```python
from build123d import *

# Parameters (mm, degrees)
BOSS_EXTRUDE1_DEPTH             = 15
H_0_266_DIAMETER_HOLE1_D        = 6.7564
SKETCH5_W                       = 1000
SKETCH5_H                       = 16
SKETCH5_W_2                     = 70
SKETCH5_H_2                     = 20.916111238
CUT_EXTRUDE1_DEPTH              = 243.332416321
BOSS_EXTRUDE4_REACH             = 242.936
SKETCH6_R                       = 3.3782
BOSS_EXTRUDE4_DIRECTION_2_REACH = 242.936


with BuildPart() as part:
    # Sketch1 → Boss-Extrude1 (new, symmetric)
    with BuildSketch(Plane.XY):
        with BuildLine():
            Line((-225, 15), (225, 15))
            ThreePointArc((225, 15), (240, 0), (225, -15))
            Line((225, -15), (-225, -15))
            ThreePointArc((-225, -15), (-240, 0), (-225, 15))
        make_face()
    extrude(amount=BOSS_EXTRUDE1_DEPTH, both=True)

    # H (0.266) Diameter Hole1 (through all)
    with Locations(Plane.XY.offset(15)):
        with Locations((-225, 0), (225, 0)):
            Hole(H_0_266_DIAMETER_HOLE1_D / 2)

    # Sketch5 → Cut-Extrude1 (cut, through all)
    with BuildSketch(Plane(origin=(0, 15, 0), x_dir=(1, 0, 0), z_dir=(0, 1, 0))):
        with Locations((-475, 0)):
            Rectangle(SKETCH5_W, SKETCH5_H)
        with Locations((210, 18.458055619)):
            Rectangle(SKETCH5_W_2, SKETCH5_H_2)
        with Locations((210, -18.458055619)):
            Rectangle(SKETCH5_W_2, SKETCH5_H_2)
    extrude(amount=-CUT_EXTRUDE1_DEPTH, mode=Mode.SUBTRACT)

    # Boss-Extrude4: up to this face of the body (flat: up to its plane)
    boss_extrude4_end = Plane(part.part.faces().sort_by_distance((-30.33914406, 0, 15))[0])
    # Sketch6 → Boss-Extrude4 (add, up to the picked face)
    with BuildSketch(Plane.XY, mode=Mode.PRIVATE) as boss_extrude4_sk1:
        with Locations((225, 0)):
            Circle(SKETCH6_R)
    boss_extrude4_tool1 = split(extrude(boss_extrude4_sk1.sketch, amount=BOSS_EXTRUDE4_REACH, mode=Mode.PRIVATE), bisect_by=boss_extrude4_end, keep=Keep.BOTH, mode=Mode.PRIVATE)
    add(boss_extrude4_tool1.solids().sort_by(Axis((225, 0, 0), (0, 0, 1)))[0])

    # Boss-Extrude4 direction 2: up to this face of the body (flat: up to its plane)
    boss_extrude4_direction_2_end = Plane(part.part.faces().sort_by_distance((-30.33914406, 0, -15))[0])
    # Sketch6 → Boss-Extrude4 direction 2 (add, up to the picked face)
    with BuildSketch(Plane.XY, mode=Mode.PRIVATE) as boss_extrude4_direction_2_sk1:
        with Locations((225, 0)):
            Circle(SKETCH6_R)
    boss_extrude4_direction_2_tool1 = split(extrude(boss_extrude4_direction_2_sk1.sketch, amount=-BOSS_EXTRUDE4_DIRECTION_2_REACH, mode=Mode.PRIVATE), bisect_by=boss_extrude4_direction_2_end, keep=Keep.BOTH, mode=Mode.PRIVATE)
    add(boss_extrude4_direction_2_tool1.solids().sort_by(Axis((225, 0, 0), (0, 0, -1)))[0])


solid = part.part
```
Can you work these out from the model? Positions are in its coordinate system, mm. A direction names the side the tool comes from. Coordinates: 2 decimals unless noted, no trailing zeros. Loops run counter-clockwise (first coordinate to the right, second up) from the corner with the lowest first, then second, coordinate; pieces in that order, holes last.
1) I need wall thicknesses on probe 1 along X at (y, z) = (-0.5, -13.5); probe 2 along Y at (x, z) = (-225, -11.5); probe 3 along Z at (x, y) = (-7, 11). Which ranges of each line are inside material? Lowest first, please.
2) Imagine slicing it at A-A on x = -12. List the corners of the cut face in (y, z) for me.
3) Thinking about a two-plate mould opening in Z: for faces 1 (the flat face through (-109, 0, -8)), 2 (the flat face through (53, -15, 0)), 3 (the flat face through (-30, 0, -15)), which applies, pulls with the +Z half, pulls with the -Z half, needs draft (parallel to the pull), parting line crosses it, or undercut?
4) Which directions (+Z, -Z, +X, -X, +Y, -Y) give clear straight access to the entire face, cutting with the end or side of a thin tool? Please do faces 4 (the flat face through (-30, 0, 15)), 5 (the flat face through (-109, 0, 8)).
5) For pin 1 (3.5 mm diameter, centred on y = -0.5, z = 11, fed in from +X); pin 2 (7.5 mm diameter, centred on y = 5, z = -12.5, fed in from +X); pin 3 (2 mm diameter, centred on x = 186.5, z = -10.5, fed in from +Y); pin 4 (1 mm diameter, centred on y = -11, z = 5, fed in from -X), each with a flat end and sliding along its axis, tell me the tip position at first contact or that it passes through.
6) Imagine slicing it at B-B on y = -8. List the corners of the cut face in (x, z) for me.
7) Imagine slicing it at C-C on z = 4. List the corners of the cut face in (x, y) for me.
8) Imagine slicing it at D-D on y = 9.5. List the corners of the cut face in (x, z) for me, plus the area to 3 significant figures.
Completed:
1. probe 1: x = -239.99 to -228.34, -221.66 to 175, 221.66 to 228.34
1. probe 2: y = -15 to -3.38, 3.38 to 15
1. probe 3: z = -15 to -8, 8 to 15
2. outline: (-15, -15) - (15, -15) - (15, -8) - (-15, -8) - close; (-15, 8) - (15, 8) - (15, 15) - (-15, 15) - close
3. face 1: undercut
3. face 2: needs draft
3. face 3: pulls with the -Z half
4. face 4: +Z, +X, -X, +Y, -Y
4. face 5: -X, +Y, -Y
5. pin 1: stops at x = 228.38
5. pin 2: stops at x = 228.14
5. pin 3: passes through
5. pin 4: stops at x = 25
6. outline: (-237.69, -15) - (175, -15) - (175, -8) - (237.69, -8) - (237.69, 8) - (175, 8) - (175, 15) - (-237.69, 15) - (-237.69, 8) - (25, 8) - (25, -8) - (-237.69, -8) - close
7. outline: (25, -15) - (225, -15) arc R15 ccw to (225, 15) - (25, 15) - close
8. outline: (-236.61, -15) - (175, -15) - (175, -8) - (236.61, -8) - (236.61, 8) - (175, 8) - (175, 15) - (-236.61, 15) - (-236.61, 8) - (25, 8) - (25, -8) - (-236.61, -8) - close
8. area: 9,150 mm2
